Autodesk Inventor part; units mm, degrees
ref_plane "YZ Plane" through (0, 0, 0) normal (1, 0, 0) x (0, 1, 0)
ref_plane "XZ Plane" through (0, 0, 0) normal (0, 1, 0) x (-1, 0, 0)
ref_plane "XY Plane" through (0, 0, 0) normal (0, 0, 1) x (1, 0, 0)
sketch "main" plane through (0, 0, 0) normal (0, 0, 1) x (1, 0, 0)
  circle A0 centre (-18.8876, -16.6215) radius 2.0828
  arc A1 (-24.8433, -18.8241) -> (-18.8876, -22.9715) centre (-18.8876, -16.6215) ccw
  line L0 (5.6124, 45.0726) -> (-28.2078, -7.9145)
  circle A2 centre (9.8531, -16.6215) radius 2.1844
  line L1 (-18.8876, -22.9715) -> (35.2506, -22.9715)
  line L2 (9.8531, 18.3035) -> (9.8531, -0.7465)
  arc A3 (9.8531, -0.7465) -> (19.3781, -10.2715) centre (19.3781, -0.7465) ccw
  circle A4 centre (9.8531, 34.1785) radius 2.1844
  line L3 (35.2481, -10.2715) -> (19.3781, -10.2715)
  arc A5 (35.2506, -22.9715) -> (35.2481, -10.2715) centre (35.2506, -16.6215) ccw
  circle A6 centre (35.2531, 34.1785) radius 2.1844
  arc A7 (35.2531, 27.8285) -> (36.6181, 40.3801) centre (35.2531, 34.1785) ccw
  circle A8 centre (35.2506, -16.6215) radius 2.1844
  line L4 (-28.3586, -9.3193) -> (-24.8433, -18.8241)
  line L5 (19.3781, 27.8285) -> (35.2531, 27.8285)
  arc A9 (19.3781, 27.8285) -> (9.8531, 18.3035) centre (19.3781, 18.3035) ccw
  arc A10 (-28.2078, -7.9145) -> (-28.3586, -9.3193) centre (-26.8697, -8.7686) ccw
  line L6 (8.9712, 46.4651) -> (36.6181, 40.3801)
  arc A11 (8.9712, 46.4651) -> (5.6124, 45.0726) centre (8.2887, 43.3643) ccw
  circle A12 centre (-3.7188, 18.6506) radius 2.0955
  circle A13 centre (-15.5942, 2.9958) radius 2.0955
  point P0 (9.379, 13.4106)
  point P1 (9.8531, 27.8285)
  dimension "d0" = 4.1656
  dimension "d1" = 12.7
  dimension "d6" = 9.525
  dimension "d9" = 1.5875
  dimension "d17" = 3.175
  dimension "d18" = 50.8
  dimension "d19" = 7.8528
  dimension "d21" = 6.35
  dimension "d22" = 36.7228
  dimension "d23" = 50.8
  dimension "d24" = 25.4
  dimension "d28" = 4.191
  dimension "d29" = 4.191
sketch "Sketch1" plane through (0, 0, 0) normal (0, 1, 0) x (-1, 0, 0)
  circle A0 centre (-54.1407, -50.8) radius 2.0828
  arc A1 (-60.0964, -53.0027) -> (-54.1407, -57.15) centre (-54.1407, -50.8) ccw
  line L0 (-29.6407, 10.894) -> (-63.461, -42.0931)
  circle A2 centre (-25.4, -50.8) radius 2.1844
  line L1 (-54.1407, -57.15) -> (-0.0025, -57.15)
  line L2 (-25.4, -15.875) -> (-25.4, -34.925)
  arc A3 (-25.4, -34.925) -> (-15.875, -44.45) centre (-15.875, -34.925) ccw
  circle A4 centre (-25.4, 0) radius 2.1844
  line L3 (-0.005, -44.45) -> (-15.875, -44.45)
  arc A5 (-0.0025, -57.15) -> (-0.005, -44.45) centre (-0.0025, -50.8) ccw
  circle A6 centre (0, 0) radius 2.1844
  arc A7 (0, -6.35) -> (1.3649, 6.2016) centre (0, 0) ccw
  circle A8 centre (-0.0025, -50.8) radius 2.1844
  line L4 (-63.6118, -43.4979) -> (-60.0964, -53.0027)
  line L5 (-15.875, -6.35) -> (0, -6.35)
  arc A9 (-15.875, -6.35) -> (-25.4, -15.875) centre (-15.875, -15.875) ccw
  arc A10 (-63.461, -42.0931) -> (-63.6118, -43.4979) centre (-62.1228, -42.9472) ccw
  line L6 (-26.2819, 12.2866) -> (1.3649, 6.2016)
  arc A11 (-26.2819, 12.2866) -> (-29.6407, 10.894) centre (-26.9644, 9.1858) ccw
  circle A12 centre (-38.9719, -15.5279) radius 2.0955
  circle A13 centre (-50.8473, -31.1828) radius 2.0955
extrude "Extrusion1" add sketch "Sketch1" along normal blind 1.5875
properties part number "Funnel Gusset V2" material "Acetal Resin, White"
Build history of the part. All positions in model axes, mm. A direction names the side the tool comes from. Coordinates: 2 decimals unless noted, no trailing zeros. Order: outer loops, then holes, each group sorted by start corner. A loop starts at its lowest first (then second) coordinate and runs counter-clockwise, first axis right, second up.
Item 1: Drill centre lines: L1, parallel to Z at x = 0, y = 0.95; L2, parallel to Z at x = 26, y = 1.15; L3, parallel to Z at x = -1, y = 0.75. Where is each one in solid material? Low to high.
Filled in:
L1: z = -57.15 to -52.98, -48.62 to -44.45, -6.35 to -2.18, 2.18 to 6.5
L2: z = -57.15 to -52.9, -48.7 to -2.1, 2.1 to 12.22
L3: z = -57.07 to -52.74, -48.86 to -44.53, -6.27 to -1.94, 1.94 to 6.28
Item 2: Saw through at A-A on z = 0. List the corners of the cut face in (x, y).
Filled in:
outline: (-6.35, 0) - (-2.18, 0) - (-2.18, 1.59) - (-6.35, 1.59) - close; (2.18, 0) - (23.22, 0) - (23.22, 1.59) - (2.18, 1.59) - close; (27.58, 0) - (36.59, 0) - (36.59, 1.59) - (27.58, 1.59) - close
Item 3: Tool access for faces 5 (the cylindrical face through (23.382, 0.783, 0.837)), 6 (the flat face through (8, 1, -44.45)): list every direction of +Z, -Z, +X, -X, +Y, -Y with a clear straight run to the whole face (end or side of a thin tool).
Filled in:
face 5: +Y, -Y
face 6: -X, +Y, -Y
Item 4: Saw through at C-C on z = -50.8. List the corners of the cut face in (x, y), then the cut area to 3 significant figures.
Filled in:
outline: (-6.35, 0) - (-2.18, 0) - (-2.18, 1.59) - (-6.35, 1.59) - close; (2.19, 0) - (23.22, 0) - (23.22, 1.59) - (2.19, 1.59) - close; (27.58, 0) - (52.06, 0) - (52.06, 1.59) - (27.58, 1.59) - close; (56.22, 0) - (60.91, 0) - (60.91, 1.59) - (56.22, 1.59) - close
area: 86.3 mm2
Item 5: Mould opens along X. For faces 1 (the cylindrical face through (-2.084, 0.783, -0.656)), 2 (the flat face through (25.4, 1, -25)), 3 (the flat face through (29, 1.588, -30)), 4 (the cylindrical face through (52.39, 0.78, -32.6)) say: released by +X, released by -X, zero draft, split by the parting line, or undercut.
Filled in:
face 1: undercut
face 2: released by -X
face 3: zero draft
face 4: undercut
Item 6: Saw through at D-D on y = 0.4. State how many separate pieces and enclosed holes the cut face has, then the cut area to 3 significant figures.
Filled in:
separate pieces: 1
enclosed holes: 7
area: 2,450 mm2
Item 7: Saw through at B-B on x = 55. List the corners of the cut face in (y, z).
Filled in:
outline: (0, -57.09) - (1.59, -57.09) - (1.59, -52.7) - (0, -52.7) - close; (0, -48.9) - (1.59, -48.9) - (1.59, -28.84) - (0, -28.84) - close
